Check sheet for the drawn part. Datum: minimum x, y, z corner. Units: mm. Give positions to 0.01 mm unless a question says otherwise; leave off trailing zeros. Write each loop counter-clockwise with the first axis right and the second up, starting at its lowest first coordinate (ties: lowest second). Pieces come first, ordered by that corner, then holes. Notation, with made-up numbers: (-27, 89) - (-12, 89) arc R18 cw to (-12, 120) - close; hole circle Ø3 at (-17, 6). An arc over 180 degrees is marked (long way). Use a Markdown table: item, result.
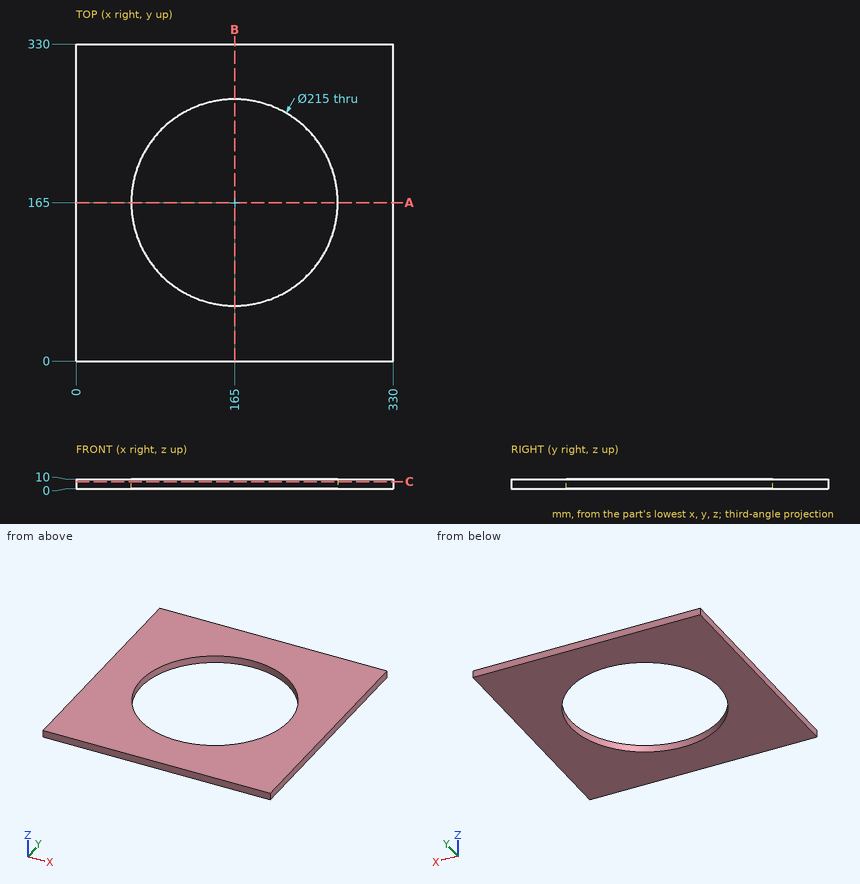
1) Section check A-A on y = 165. Record the boundary of the cut face in (x, z).
Working result:
| item | result |
|---|---|
| outline | (0, 0) - (57.5, 0) - (57.5, 10) - (0, 10) - close; (272.5, 0) - (330, 0) - (330, 10) - (272.5, 10) - close |
2) Depth check by flat-ended pin: P1, Ø3, axis at x = 85, z = 1, coming from the -Y side; P2, Ø3, axis at x = 91, y = 238.5, coming from the +Z side. Enter the tip coordinate at first touch or a pass-through.
Working result:
| item | result |
|---|---|
| P1 | stops at y = 0 |
| P2 | passes through |
3) Material ranges on L1, parallel to Y at x = 165, z = 7; L2, parallel to X at y = 132, z = 2.5; L3, parallel to X at y = 230.5, z = 7.5, recorded low to high. Write a range as from..to.
Working result:
| item | result |
|---|---|
| L1 | y = 0..57.5, 272.5..330 |
| L2 | x = 0..62.69, 267.31..330 |
| L3 | x = 0..79.76, 250.24..330 |
4) Section check C-C on z = 7.25. Record the boundary of the cut face in (x, y), then the cut area to 3 significant figures.
Working result:
| item | result |
|---|---|
| outline | (0, 0) - (330, 0) - (330, 330) - (0, 330) - close; hole circle Ø215 at (165, 165) |
| area | 72,600 mm² |
